Geometry: final body of the model. Coordinates: model frame, mm. Coordinates: 2 decimals unless noted, no trailing zeros. Write each loop counter-clockwise with the first axis right and the second up, starting at its lowest first coordinate (ties: lowest second). Pieces come first, ordered by that corner, then holes.
from build123d import *

# Parameters (mm, degrees)
F0_W     = 40
F0_H     = 300
F0_H_2   = 25
F0_H_3   = 65
F1_DEPTH = 25
F2_D     = 10


with BuildPart() as f1:
    # F0 (on Front) → F1 (new body)
    with BuildSketch(Plane.XZ):
        with Locations((-20, 20)):
            Rectangle(F0_W, F0_H)
        with Locations((20, 20)):
            Rectangle(F0_W, F0_H)
        with Locations((20, 182.5)):
            Rectangle(F0_W, F0_H_2)
        with Locations((-20, 182.5)):
            Rectangle(F0_W, F0_H_2)
        with Locations((20, -162.5)):
            Rectangle(F0_W, F0_H_3)
        with Locations((-20, -162.5)):
            Rectangle(F0_W, F0_H_3)
    extrude(amount=-F1_DEPTH)

    # F2 (through all)
    with Locations(Plane.XZ):
        with Locations((0, 170), (0, -130)):
            Hole(F2_D / 2)


solid = f1.part
Item 1: Pull-direction query (Z, two-part tool) for faces 1 (the flat face through (40, 12, -3)), 2 (the cylindrical face through (0.651, 12.675, 174.957)), 3 (the flat face through (1, 12, 195)); classes: released by +Z, released by -Z, zero draft, split by the parting line, or undercut.
Derived:
face 1: zero draft
face 2: undercut
face 3: released by +Z
Item 2: Section A-A, the plane z = 170. Output: boundary loops of the cut face in (x, y).
Derived:
outline: (-40, 0) - (-5, 0) - (-5, 25) - (-40, 25) - close; (5, 0) - (40, 0) - (40, 25) - (5, 25) - close
Item 3: Material intervals for probe 1 along Z at (x, y) = (0, 14.75), sorted ascending.
Derived:
probe 1: z = -195 to -135, -125 to 165, 175 to 195
Item 4: Section B-B, the plane x = 0. Output: boundary loops of the cut face in (y, z), plus the area to 3 significant figures.
Derived:
outline: (0, -195) - (25, -195) - (25, -135) - (0, -135) - close; (0, -125) - (25, -125) - (25, 165) - (0, 165) - close; (0, 175) - (25, 175) - (25, 195) - (0, 195) - close
area: 9,250 mm2
